Work out the finished part from the listing and answer in its coordinate system (mm). A direction names the side the tool comes from. Round coordinates to 2 decimals unless told otherwise and drop trailing zeros. Order: outer loops, then holes, each group sorted by start corner. A loop starts at its lowest first (then second) coordinate and runs counter-clockwise, first axis right, second up. Notation, with made-up numbers: (35, 17.5) -> (70, 17.5) arc R15 cw to (70, 33.5) -> close; hole circle Ø4 at (58, 74.5). An arc over 180 degrees is marked (long way). Use one line per item in the form item = value.
```python
from build123d import *

# Parameters (mm, degrees)
F0_W     = 127
F0_H     = 76.2
F1_DEPTH = 50.8
F2_W     = 38.1
F2_H     = 38.1
F3_DEPTH = 25.4
F4_SIZE  = 5.08


with BuildPart() as f1:
    # F0 (on Front) → F1 (new body)
    with BuildSketch(Plane.XZ):
        with Locations((-5.314695, -11.454906)):
            Rectangle(F0_W, F0_H)
    extrude(amount=F1_DEPTH)

    # F2 (on face) → F3 (cut)
    with BuildSketch(Plane.XZ.offset(50.8)):
        with Locations((-5.314695, -11.454906)):
            Rectangle(F2_W, F2_H)
    extrude(amount=-F3_DEPTH, mode=Mode.SUBTRACT)

    # F4
    f4_edges = [f1.edges().sort_by_distance(p)[0] for p in [
        (-5.314695, -50.8, 26.645094),
        (58.185305, -50.8, -11.454906),
        (-5.314695, -50.8, -49.554906),
        (-68.814695, -50.8, -11.454906),
    ]]
    chamfer(f4_edges, length=F4_SIZE)


solid = f1.part
```
Item 1: The part is cut by section C-C, the plane x = 5. Give the vertices of the cut face in (y, z), and give its area (3 significant figures).
Findings:
outline = (-50.8, -44.47) -> (-45.72, -49.55) -> (0, -49.55) -> (0, 26.65) -> (-45.72, 26.65) -> (-50.8, 21.57) -> (-50.8, 7.6) -> (-25.4, 7.6) -> (-25.4, -30.5) -> (-50.8, -30.5) -> close
area = 2,880 mm^2
Item 2: Determine the mould class of faces 3 (the flat face through (-6, -38, 7.595)), 4 (the flat face through (-6, -23, -49.555)), 5 (the flat face through (-68.815, -23, -12)), 6 (the flat face through (13.735, -38, -12)) for opening direction Z: released by +Z, released by -Z, zero draft, split by the parting line, or undercut.
Findings:
face_3 = undercut
face_4 = released by -Z
face_5 = zero draft
face_6 = undercut
Item 3: For faces 1 (the flat face through (-6.204, -48.296, -46.979)), 2 (the flat face through (-6, -38, -30.505)), determine the directions among +Z, -Z, +X, -X, +Y, -Y from which every point of the face is accessible in a straight line to the end or side of a thin tool.
Findings:
face_1 = -Z, +X, -X, -Y
face_2 = -Y
Item 4: A flat-ended cylindrical pin translates along its axis: P1, Ø19, axis at x = -4, z = -10.5, coming from the -Y side. Find the tip coordinate at first contact, or state that the pin passes through.
Findings:
P1 = -25.4
Item 5: The part is cut by section B-B, the plane z = -21.5. Give the vertices of the cut face in (x, y).
Findings:
outline = (-68.81, -45.72) -> (-63.73, -50.8) -> (-24.36, -50.8) -> (-24.36, -25.4) -> (13.74, -25.4) -> (13.74, -50.8) -> (53.11, -50.8) -> (58.19, -45.72) -> (58.19, 0) -> (-68.81, 0) -> close
Item 6: Consider line 1 along Z through (x, y) = (2, -25.5); line 2 along X through (y, z) = (-45, 4); line 3 along Y through (x, z) = (2.5, -26). Determine where each line is inside the solid, lowest interval first.
Findings:
line_1 = -49.55 to -30.5, 7.6 to 26.65
line_2 = -68.81 to -24.36, 13.74 to 58.19
line_3 = -25.4 to 0
Item 7: The part is cut by section A-A, the plane y = -41.5. Give the vertices of the cut face in (x, z), and give its area (3 significant figures).
Findings:
outline = (-68.81, -49.55) -> (58.19, -49.55) -> (58.19, 26.65) -> (-68.81, 26.65) -> close; hole (-24.36, -30.5) -> (13.74, -30.5) -> (13.74, 7.6) -> (-24.36, 7.6) -> close
area = 8,230 mm^2
